from build123d import *

# Parameters (mm, degrees)
BOSS_EXTRUDE1_DEPTH   = 10
FILLET1_R             = 1
F_4_CLEARANCE_HOLE1_D = 3.2639


with BuildPart() as part:
    # Sketch1 → Boss-Extrude1 (new body)
    with BuildSketch(Plane.XY):
        with BuildLine():
            Line((-20.875, 0), (-20.875, -20))
            Line((-20.875, -20), (-32.875, -20))
            Line((-32.875, -20), (-32.875, -25.72))
            Line((-32.875, -25.72), (-6, -25.72))
            Line((-6, -25.72), (-6, -14.69747002))
            ThreePointArc((-6, -14.69747002), (0, 15.875), (6, -14.69747002))
            Line((6, -14.69747002), (6, -25.72))
            Line((6, -25.72), (32.875, -25.72))
            Line((32.875, -25.72), (32.875, -20))
            Line((32.875, -20), (20.875, -20))
            Line((20.875, -20), (20.875, 0))
            ThreePointArc((20.875, 0), (0, 20.875), (-20.875, 0))
        make_face()
    extrude(amount=BOSS_EXTRUDE1_DEPTH)

    # Fillet1
    fillet1_edges = [part.edges().sort_by_distance(p)[0] for p in [
        (-32.875, -22.86, 0),
        (32.875, -22.86, 0),
        (32.875, -22.86, 10),
        (-32.875, -22.86, 10),
    ]]
    fillet(fillet1_edges, radius=FILLET1_R)

    # #4 Clearance Hole1 (through all)
    with Locations(Plane(origin=(0, -20, 0), x_dir=(1, 0, 0), z_dir=(0, 1, 0))):
        with Locations((-26.875, -5), (26.875, -5)):
            Hole(F_4_CLEARANCE_HOLE1_D / 2)


solid = part.part
Check sheet for the modelled part. Datum: model origin and axes. Units: mm. A direction names the side the tool comes from. Round coordinates to 2 decimals unless told otherwise and drop trailing zeros. Loops run counter-clockwise (first coordinate to the right, second up) from the corner with the lowest first, then second, coordinate; pieces in that order, holes last. Notation, with made-up numbers: M 5.25,17.5 L 9.25,17.5 A9 ccw 9.25,29.5 Z; hole C 88.25,-19.75 d8. An arc over 180 degrees is marked long. One line per item, written item: value.
(1) Release check for a two-part mould opening along Z. For faces 1 (the face through (7, -16, 0)), 2 (the face through (-25.245, -22.9, 4.928)), 3 (the face through (-32.875, -23, 5)), 4 (the face through (7, -16, 10)) record: +Z half, -Z half, draft (parallel to the pull), parting line (faces both ways), or undercut.
Computed values:
face 1: -Z half
face 2: undercut
face 3: draft
face 4: +Z half
(2) Sectioned sample at A-A, the plane y = -21.5. Record the cut outline in (x, z) (3 decimals).
Computed values:
outline: M -32.875,1 A1 ccw -31.875,0 L -6,0 L -6,10 L -31.875,10 A1 ccw -32.875,9 Z; M 6,0 L 31.875,0 A1 ccw 32.875,1 L 32.875,9 A1 ccw 31.875,10 L 6,10 Z; hole C -26.875,5 d3.264; hole C 26.875,5 d3.264
(3) Sectioned sample at D-D, the plane y = 8. Record the cut outline in (x, z), then the cut area to 3 significant figures.
Computed values:
outline: M -19.28,0 L -13.71,0 L -13.71,10 L -19.28,10 Z; M 13.71,0 L 19.28,0 L 19.28,10 L 13.71,10 Z
area: 111 mm^2
(4) Sectioned sample at C-C, the plane x = 7. Record the cut outline in (y, z), then the cut area to 3 significant figures.
Computed values:
outline: M -25.72,0 L -14.25,0 L -14.25,10 L -25.72,10 Z; M 14.25,0 L 19.67,0 L 19.67,10 L 14.25,10 Z
area: 169 mm^2
(5) Thickness scan on line 1 (X direction, y = -22.15, z = 5) (3 decimals); line 2 (X direction, y = -6, z = 1.75) (3 decimals); line 3 (Y direction, x = 10, z = 6.5). Record the ranges inside material, lowest first.
Computed values:
line 1: x = -32.875 to -28.507, -25.243 to -6, 6 to 25.243, 28.507 to 32.875
line 2: x = -20.875 to -14.697, 14.697 to 20.875
line 3: y = -25.72 to -12.33, 12.33 to 18.32
(6) Depth check by flat-ended pin: pin 1 Ø3 at (x, z) = (-26.875, 5) entering from -Y; pin 2 Ø5 at (x, z) = (26.875, 5) entering from +Y; pin 3 Ø3 at (y, z) = (-1.5, 6.5) entering from +X (3 decimals); pin 4 Ø4 at (y, z) = (-3, 1.5) entering from -X (3 decimals). Enter the tip coordinate at first touch or a pass-through.
Computed values:
pin 1: passes through
pin 2: stops at y = -20
pin 3: stops at x = 20.875
pin 4: stops at x = -20.875
(7) Sectioned sample at B-B, the plane z = 5. Record the cut outline in (x, y) (3 decimals).
Computed values:
outline: M -32.875,-25.72 L -28.507,-25.72 L -28.507,-20 L -32.875,-20 Z; M -25.243,-25.72 L -6,-25.72 L -6,-14.697 A15.875 cw long 6,-14.697 L 6,-25.72 L 25.243,-25.72 L 25.243,-20 L 20.875,-20 L 20.875,0 A20.875 ccw -20.875,0 L -20.875,-20 L -25.243,-20 Z; M 28.507,-25.72 L 32.875,-25.72 L 32.875,-20 L 28.507,-20 Z
(8) Access from +Z, -Z, +X, -X, +Y, -Y to the whole of each face (thin tool, end or side, straight path). Record for faces 5 (the face through (19, -25.72, 5)), 6 (the face through (20.875, -10, 5)), 7 (the face through (0.46, 20.87, 4.93)), 8 (the face through (-6, -20, 5)), 9 (the face through (-25, -20, 4)).
Computed values:
face 5: +Z, -Z, +X, -X, -Y
face 6: +Z, -Z, +X, +Y
face 7: +Z, -Z, +Y
face 8: +Z, -Z, -Y
face 9: +Z, -Z, -X, +Y
